Check sheet for the modelled part. Datum: model origin and axes. Units: mm. Face numbers are marked on the shaded views. Round coordinates to 2 decimals unless told otherwise and drop trailing zeros. Order: outer loops, then holes, each group sorted by start corner. A loop starts at its lowest first (then second) coordinate and runs counter-clockwise, first axis right, second up.
Q1. Cross-section at A-A on y = -15.5. Record the cut outline in (x, z) (3 decimals), then the cut area to 3 significant figures.
Q2. Cross-section at C-C on x = -15.5. Record the cut outline in (y, z), then the cut area to 3 significant figures.
Q3. Cross-section at B-B on x = 0. Record the cut outline in (y, z).
Q4. Cross-section at D-D on y = 0. Record the cut outline in (x, z) (3 decimals).
Q5. Depth check by flat-ended pin: P1, Ø12, axis at x = 46.5, z = -13, coming from the +Y side; P2, Ø2.5, axis at x = -9, z = -0.5, coming from the +Y side; P3, Ø7.5, axis at x = -33.5, y = 4.5, coming from the -Z side (3 decimals); P4, Ø3, axis at y = -23, z = -12.5, coming from the -X side. Enter the tip coordinate at first touch or a pass-through.
Q6. Mould release check, pull along X, two halves, no side actions. Record for the marked faces 1, 2, 3 and 4: +X half, -X half, draft (parallel to the pull), parting line (faces both ways), or undercut.
Q7. Scan lines: probe 1 along Y at (x, z) = (15.5, 2.5); probe 2 along Z at (x, y) = (-36, 25.5) (3 decimals); probe 3 along X at (y, z) = (-11, -0.25). Record each from-to range of solid material in increasing order.
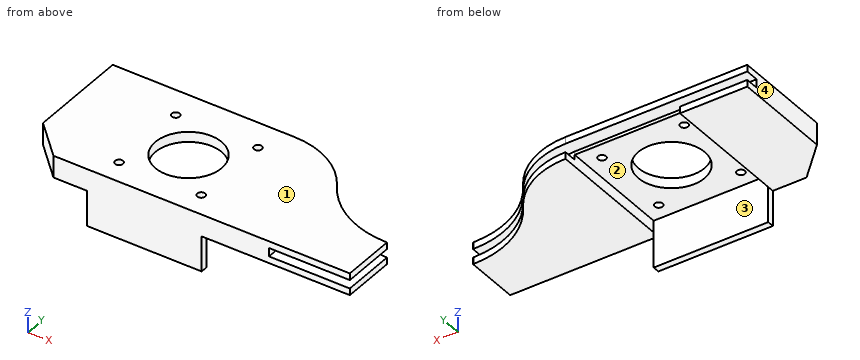
Autodesk Inventor part; units mm, degrees
ref_plane "YZ Plane" through (0, 0, 0) normal (1, 0, 0) x (0, 1, 0)
ref_plane "XZ Plane" through (0, 0, 0) normal (0, 1, 0) x (-1, 0, 0)
ref_plane "XY Plane" through (0, 0, 0) normal (0, 0, 1) x (1, 0, 0)
sketch "Sketch1" plane through (0, 0, 0) normal (0, 0, 1) x (1, 0, 0)
  circle A0 centre (0, 0) radius 12.5
  line L0 (0, 0) -> (15.5, 0)
  line L1 (0, 0) -> (15.5, 0) construction
  line L2 (15.5, 0) -> (15.5, 15.5)
  circle A1 centre (15.5, 15.5) radius 1.5
  circle A2 centre (-15.5, 15.5) radius 1.5
  circle A3 centre (15.5, -15.5) radius 1.5
  circle A4 centre (-15.5, -15.5) radius 1.5
  line L3 (21.59, -21.59) -> (-21.59, -21.59)
  line L4 (-21.59, -21.59) -> (-21.59, 21.59)
  line L5 (-21.59, 21.59) -> (21.59, 21.59)
  line L6 (21.59, 21.59) -> (21.59, -21.59)
  line L7 (21.59, -21.59) -> (-21.59, 21.59) construction
  line L8 (-21.59, -21.59) -> (21.59, 21.59) construction
  dimension "d0" = 25
  dimension "d1" = 15.5
  dimension "d2" = 0
  dimension "d3" = 15.5
  dimension "d4" = 3
  dimension "d7" = 31
  dimension "d10" = 31
  dimension "d13" = 43.18
  dimension "d14" = 43.18
extrude "Extrusion1" add sketch "Sketch1" along normal blind 3.81
sketch "Sketch2" plane through (-21.59, -21.59, 0) normal (0, -1, 0) x (1, 0, 0)
  line L0 (0, 3.81) -> (43.18, 3.81)
  line L1 (0, 3.81) -> (43.18, 3.81)
  line L2 (43.18, 3.81) -> (43.18, -17.78)
  line L3 (43.18, -17.78) -> (0, -17.78)
  line L4 (0, -17.78) -> (0, 3.81)
  point P0 (21.59, 0)
  dimension "d17" = 21.59
extrude "Extrusion2" add sketch "Sketch2" along normal blind 2.54
sketch "Sketch3" plane through (0, 0, 3.81) normal (0, 0, 1) x (1, 0, 0)
  line L0 (-21.59, 21.59) -> (21.59, 21.59)
  circle A0 centre (0, 0) radius 12.5
  circle A1 centre (-15.5, -15.5) radius 1.5
  circle A2 centre (15.5, -15.5) radius 1.5
  circle A3 centre (-15.5, 15.5) radius 1.5
  circle A4 centre (15.5, 15.5) radius 1.5
  line L1 (21.59, 21.59) -> (21.59, -24.13)
  line L2 (21.59, 21.59) -> (-21.59, 21.59)
  line L3 (-21.59, 21.59) -> (-21.59, -24.13)
  line L4 (21.59, -24.13) -> (-21.59, -24.13)
  line L5 (-21.59, 26.67) -> (21.59, 26.67)
  arc A5 (52.07, -3.81) -> (21.59, 26.67) centre (21.59, -3.81) ccw
  line L6 (52.07, -3.81) -> (52.07, -24.13)
  line L7 (-21.59, 26.67) -> (-21.59, 21.59)
  line L8 (-21.59, 21.59) -> (21.59, 21.59)
  line L9 (21.59, 21.59) -> (21.59, -21.59)
  line L10 (21.59, 21.59) -> (21.59, -24.13)
  line L11 (21.59, 21.59) -> (21.59, -24.13)
  line L12 (21.59, -24.13) -> (52.07, -24.13)
extrude "Extrusion3" add sketch "Sketch3" against normal blind 2.54 contours L7 L5 A5 L6 L12 L1 L0
sketch "Sketch4" plane through (0, 0, 1.27) normal (0, 0, -1) x (-1, 0, 0)
  line L0 (-21.59, 21.59) -> (-21.59, -24.13)
  line L1 (-21.59, -24.13) -> (-46.99, -24.13)
  arc A0 (-21.59, 26.67) -> (-52.07, -3.81) centre (-21.59, -3.81) ccw
  arc A1 (-21.59, 21.59) -> (-46.99, -3.81) centre (-21.59, -3.81) ccw
  line L2 (-46.99, -3.81) -> (-46.99, -24.13)
  line L3 (-21.59, 21.59) -> (-21.59, -24.13)
  line L4 (-21.59, 21.59) -> (-21.59, -24.13)
  line L5 (-21.59, -24.13) -> (-21.59, 21.59)
  point P0 (0, 0)
  dimension "d26" = 25.4
  dimension "d27" = 5.08
extrude "Extrusion4" add sketch "Sketch4" along normal blind 3.175
sketch "Sketch5" plane through (0, 0, -1.905) normal (0, 0, -1) x (-1, 0, 0)
  line L0 (-46.99, -24.13) -> (-46.99, -3.81)
  arc A0 (-21.59, 21.59) -> (-46.99, -3.81) centre (-21.59, -3.81) ccw
  line L1 (21.59, 21.59) -> (-21.59, 21.59)
  line L2 (21.59, 21.59) -> (21.59, 26.67)
  line L3 (21.59, 26.67) -> (-21.59, 26.67)
  arc A1 (-21.59, 26.67) -> (-52.07, -3.81) centre (-21.59, -3.81) ccw
  line L4 (-52.07, -3.81) -> (-52.07, -24.13)
  line L5 (-52.07, -24.13) -> (-46.99, -24.13)
  line L6 (-21.59, -21.59) -> (-21.59, -24.13)
  line L7 (-21.59, -21.59) -> (-21.59, 21.59)
  arc A2 (-21.59, 21.59) -> (-46.99, -3.81) centre (-21.59, -3.81) ccw
  line L8 (-46.99, -3.81) -> (-46.99, -24.13)
  line L9 (-46.99, -24.13) -> (-21.59, -24.13)
  line L10 (21.59, 21.59) -> (-21.59, 21.59)
  line L11 (-21.59, 21.59) -> (-21.59, 26.67)
  point P0 (0, 0)
extrude "Extrusion5" add sketch "Sketch5" along normal blind 2.54 contours L5 L4 A1 L11 A0 L0 | L0 A0 L7 L6 L9
sketch "Sketch6" plane through (-21.59, -21.59, 0) normal (-1, 0, 0) x (0, 0, 1)
  line L0 (0, 43.18) -> (0, 0)
  line L1 (0, 43.18) -> (-1.905, 43.18)
  line L2 (-1.905, 43.18) -> (-1.905, 48.26)
  line L3 (-1.905, 48.26) -> (-4.445, 48.26)
  line L4 (-4.445, 0) -> (-4.445, 48.26)
  line L5 (0, 0) -> (-4.445, 0)
  line L6 (1.27, 17.78) -> (1.27, 43.18)
  line L7 (0, 0) -> (0, 43.18)
  line L8 (-17.78, 0) -> (0, 0)
  line L9 (-17.78, 0) -> (-17.78, -2.54)
  line L10 (3.81, -2.54) -> (-17.78, -2.54)
  line L11 (3.81, 48.26) -> (3.81, -2.54)
  line L12 (3.81, 48.26) -> (1.27, 48.26)
  line L13 (1.27, 43.18) -> (1.27, 48.26)
  line L14 (0, 43.18) -> (1.27, 43.18)
  line L15 (-4.445, 0) -> (-17.78, 0)
  line L16 (-17.78, -2.54) -> (-4.445, -2.54)
  line L17 (-4.445, 0) -> (-4.445, -2.54)
  point P0 (0, 21.59)
extrude "Extrusion6" add sketch "Sketch6" along normal blind 25.4 contours L14 L13 L12 L11 L10 L17 L5 L0 | L0 L5 L4 L3 L2 L1
sketch "Sketch7" plane through (52.07, -24.13, -1.905) normal (1, 0, 0) x (0, 0, -1)
  line L0 (0, 20.32) -> (0, 0)
  line L1 (0, 0) -> (2.54, 0)
  line L2 (2.54, 20.32) -> (2.54, 0)
  line L3 (0, 20.32) -> (2.54, 20.32)
  line L4 (-5.715, 0) -> (-5.715, 20.32)
  line L5 (-5.715, 0) -> (-3.175, 0)
  line L6 (-3.175, 20.32) -> (-3.175, 0)
  line L7 (-5.715, 20.32) -> (-3.175, 20.32)
  point P0 (-1.905, 24.13)
extrude "Extrusion7" add sketch "Sketch7" along normal blind 25.4
fillet "Fillet1" radius 34.925 2 edges at (52.07, -3.81, 2.54) (52.07, -3.81, -3.175)
chamfer "Chamfer1" distance 12.7 angle 45 1 edges at (-46.99, -24.13, -0.3175)
properties part number "RemoteExtruderV4"
Results found:
1. outline: (-42.92, -4.445) - (-21.59, -4.445) - (-21.59, 0) - (-17, 0) - (-17, 3.81) - (-42.92, 3.81) - close; (-14, 0) - (14, 0) - (14, 3.81) - (-14, 3.81) - close; (17, 0) - (21.59, 0) - (21.59, -4.445) - (77.47, -4.445) - (77.47, -1.905) - (46.99, -1.905) - (46.99, 1.27) - (77.47, 1.27) - (77.47, 3.81) - (17, 3.81) - close
1. area: 682 mm2
2. outline: (-24.13, -17.78) - (-21.59, -17.78) - (-21.59, 0) - (-17, 0) - (-17, 3.81) - (-24.13, 3.81) - close; (-14, 0) - (14, 0) - (14, 3.81) - (-14, 3.81) - close; (17, 0) - (21.59, 0) - (21.59, 1.27) - (26.67, 1.27) - (26.67, 3.81) - (17, 3.81) - close
2. area: 209 mm2
3. outline: (-24.13, -17.78) - (-21.59, -17.78) - (-21.59, 0) - (-12.5, 0) - (-12.5, 3.81) - (-24.13, 3.81) - close; (12.5, 0) - (21.59, 0) - (21.59, 1.27) - (26.67, 1.27) - (26.67, 3.81) - (12.5, 3.81) - close
4. outline: (-46.99, -4.445) - (-21.59, -4.445) - (-21.59, 0) - (-12.5, 0) - (-12.5, 3.81) - (-46.99, 3.81) - close; (12.5, 0) - (21.59, 0) - (21.59, -4.445) - (61.027, -4.445) - (61.027, -1.905) - (46.703, -1.905) - (46.703, 1.27) - (61.027, 1.27) - (61.027, 3.81) - (12.5, 3.81) - close
5. P1: passes through
5. P2: stops at y = 21.59
5. P3: stops at z = -4.445
5. P4: stops at x = -21.59
6. face 1: draft
6. face 2: undercut
6. face 3: undercut
6. face 4: -X half
7. probe 1: y = -24.13 to -17, -14 to 14, 17 to 26.67
7. probe 2: z = -4.445 to -1.905, 1.27 to 3.81
7. probe 3: x = -46.99 to -21.59, 21.59 to 46.99
